from build123d import *

# Parameters (mm, degrees)
F0_W     = 508
F0_H     = 508
F1_DEPTH = 25
F3_DEPTH = 25
F5_W     = 60
F5_H     = 160
F6_DEPTH = 25


with BuildPart() as f1:
    # F0 (on Top) → F1 (new body)
    with BuildSketch(Plane.XY):
        Rectangle(F0_W, F0_H)
    extrude(amount=-F1_DEPTH)

    # F2 (on face) → F3 (join)
    with BuildSketch(Plane(origin=(-254, 0, 0), x_dir=(0, -1, 0), z_dir=(-1, 0, 0))):
        Polygon((254, -25), (194, -25), (286.3760430703, -185), (346.3760430703, -185), align=None)
    extrude(amount=-F3_DEPTH)

    # F4: F1 across plane


with BuildPart() as f1_1:
    add(f1.part)
    add(f1.part.mirror(Plane.YZ))

    # F5 (on face) → F6 (join)
    with BuildSketch(Plane(origin=(0, 254, 0), x_dir=(-1, 0, 0), z_dir=(0, 1, 0))):
        with Locations((-224, -105)):
            Rectangle(F5_W, F5_H)
        with Locations((224, -105)):
            Rectangle(F5_W, F5_H)
    extrude(amount=-F6_DEPTH)


solid = f1_1.part
Can you work these out from the model? Positions are in its coordinate system, mm. A direction names the side the tool comes from. Coordinates: 2 decimals unless noted, no trailing zeros. Order: outer loops, then holes, each group sorted by start corner. A loop starts at its lowest first (then second) coordinate and runs counter-clockwise, first axis right, second up. Notation, with made-up numbers: (50, 71) - (90, 71) arc R25 cw to (90, 108) - close; hole circle Ø8 at (34, 19.5). An arc over 180 degrees is marked (long way). Answer as a JSON object with one key per item and string values. Group by question number.
Q1. Imagine slicing it at C-C (x = 207). Please give me the cut outline in (y, z), and give its area (3 significant figures).
Q2. I need wall thicknesses on line 1 (Z direction, x = 224, y = 108); line 2 (X direction, y = -279, z = -100); line 3 (Y direction, x = -73, z = -16). Which ranges of each line are inside material? Lowest first, please. Write a range as from..to.
Q3. We'd pull the mould along X, two halves only. Please class faces 6 (the face through (229, -269, -104)), 7 (the face through (-241.68, -239.54, -103.88)), 8 (the face through (-254, -67, -24)): +X half, -X half, draft (parallel to the pull), parting line (faces both ways), or undercut.
Q4. On a 3-axis mill with a long thin cutter (end or side, diameter ignored), from which of +Z, -Z, +X, -X, +Y, -Y can I reach the whole of each face in a straight line? I mean faces 1 (the face through (194, 242, -106)), 2 (the face through (-241.675, -300.835, -106.12)), 3 (the face through (241.68, -239.54, -103.88)), 4 (the face through (-229, -269, -104)), 5 (the face through (224, 242, -185)). Say none if no direction works.
Q5. Imagine slicing it at B-B (y = -294.5). Please give me the cut outline in (x, z).
Q6. Imagine slicing it at A-A (z = -117.5). Please give me the cut outline in (x, y).
Q7. Imagine slicing it at D-D (y = -156.5). Please give me the cut outline in (x, z).
Q8. Will these pins go through, and if not, where does the flat tip stop? P1, Ø12, axis at x = -162.5, y = -20, coming from the -Z side; P2, Ø20, axis at x = 94, z = -7.5, coming from the -Y side; P3, Ø18, axis at x = -238, z = -96, coming from the -Y side.
Determined:
{
 "1": {"outline": "(-254, -25) - (229, -25) - (229, -185) - (254, -185) - (254, 0) - (-254, 0) - close", "area": "16,700 mm2"},
 "2": {"line 1": "z = -25..0", "line 2": "x = -254..-229, 229..254", "line 3": "y = -254..254"},
 "3": {"face 6": "undercut", "face 7": "draft", "face 8": "-X half"},
 "4": {"face 1": "-Z, +Y, -Y", "face 2": "+Z, +X, -X, -Y", "face 3": "-Z, +X, -X", "face 4": "-Z, -Y", "face 5": "-Z, +X, -X, +Y, -Y"},
 "5": {"outline": "(-254, -185) - (-229, -185) - (-229, -95.15) - (-254, -95.15) - close; (229, -185) - (254, -185) - (254, -95.15) - (229, -95.15) - close"},
 "6": {"outline": "(-254, -307.4) - (-229, -307.4) - (-229, -247.4) - (-254, -247.4) - close; (-254, 229) - (-194, 229) - (-194, 254) - (-254, 254) - close; (194, 229) - (254, 229) - (254, 254) - (194, 254) - close; (229, -307.4) - (254, -307.4) - (254, -247.4) - (229, -247.4) - close"},
 "7": {"outline": "(-254, -25) - (254, -25) - (254, 0) - (-254, 0) - close"},
 "8": {"P1": "stops at z = -25", "P2": "stops at y = -254", "P3": "stops at y = -300.19"}
}
